```python
from build123d import *

# Parameters (mm, degrees)
F0_R     = 14.75
F1_DEPTH = 20
F3_DEPTH = 17.53955
F4_DEPTH = 74
F6_DEPTH = 19
F7_W     = 3.96875
F7_H     = 17.4625
F8_DEPTH = 20.001


with BuildPart() as f1:
    # F0 (on Top) → F1 (new body)
    with BuildSketch(Plane.XY):
        Circle(F0_R)
    extrude(amount=F1_DEPTH)

    # F2 (on face) → F3 (join)
    with BuildSketch(Plane(origin=(0, 0, 0), x_dir=(1, 0, 0), z_dir=(0, 0, -1))):
        with BuildLine():
            Line((0, -14.75), (0, -17.8051246337))
            Line((0, -17.8051246337), (14.75, -17.8051246337))
            Line((14.75, -17.8051246337), (14.75, 0))
            ThreePointArc((14.75, 0), (10.4298250225, -10.4298250225), (0, -14.75))
        make_face()
        with BuildLine():
            Line((-14.75, -17.8051246337), (0, -17.8051246337))
            Line((0, -17.8051246337), (0, -14.75))
            ThreePointArc((0, -14.75), (-10.4298250225, -10.4298250225), (-14.75, 0))
            Line((-14.75, 0), (-14.75, -17.8051246337))
        make_face()
        with BuildLine():
            ThreePointArc((-14.75, 0), (-10.4298250225, -10.4298250225), (0, -14.75))
            Line((0, -14.75), (0, 0))
            Line((0, 0), (-14.75, 0))
        make_face()
        with BuildLine():
            Line((0, 0), (0, -14.75))
            ThreePointArc((0, -14.75), (10.4298250225, -10.4298250225), (14.75, 0))
            Line((14.75, 0), (0, 0))
        make_face()
        Polygon((14.75, -17.8051246337), (0, -17.8051246337), (-14.75, -17.8051246337), (-14.75, -37.8051246337), (14.75, -37.8051246337), align=None)
    extrude(amount=-F3_DEPTH)

    # F2 (on face) → F4 (join)
    with BuildSketch(Plane(origin=(0, 0, 0), x_dir=(1, 0, 0), z_dir=(0, 0, -1))):
        Polygon((14.75, -17.8051246337), (0, -17.8051246337), (-14.75, -17.8051246337), (-14.75, -37.8051246337), (14.75, -37.8051246337), align=None)
    extrude(amount=F4_DEPTH)

    # F5 (on face) → F6 (cut)
    with BuildSketch(Plane.XY.offset(20)):
        with BuildLine():
            Line((2, -1.5), (2, 1.5))
            ThreePointArc((2, 1.5), (-2.5, 0), (2, -1.5))
        make_face()
    extrude(amount=-F6_DEPTH, mode=Mode.SUBTRACT)

    # F7 (on face) → F8 (cut, through all)
    with BuildSketch(Plane.XZ.offset(-17.8051246337)):
        with Locations((5.159375, -34.33125)):
            Rectangle(F7_W, F7_H)
        with Locations((-5.159375, -34.33125)):
            Rectangle(F7_W, F7_H)
    extrude(amount=-F8_DEPTH, mode=Mode.SUBTRACT)


solid = f1.part
```
Could you check a few things on this model? Use its own coordinates, in mm. A direction names the side the tool comes from. Give positions to 0.01 mm unless a question says otherwise; leave off trailing zeros. Write each loop counter-clockwise with the first axis right and the second up, starting at its lowest first coordinate (ties: lowest second). Pieces come first, ordered by that corner, then holes. Notation, with made-up numbers: (-39, -14) - (4, -14) arc R27 cw to (4, 2) - close; hole circle Ø8 at (69.25, -18). An arc over 180 degrees is marked (long way). One line per item, written item: value. Start each with the question number.
Item 1: Imagine slicing it at C-C, the plane x = 0. List the corners of the cut face in (y, z) for me, and give its area (3 significant figures).
Item 2: I'm going to push flat-ended pins straight in: pin 1 (10 mm diameter, centred on x = 4.5, z = 8.5, fed in from -Y); pin 2 (1 mm diameter, centred on x = -4, y = 24.5, fed in from +Z); pin 3 (6 mm diameter, centred on x = 4.5, z = -59.5, fed in from -Y); pin 4 (5 mm diameter, centred on y = -3.5, z = -4.5, fed in from +X). Where does each tip first touch, or does it pass through?
Item 3: Imagine slicing it at A-A, the plane z = -30. List the corners of the cut face in (x, y) for me (3 decimals).
Item 4: If we mould it in two halves opening along Z, with no side actions, what happens to faces 4 (the face through (-3.175, 28, -34)), 5 (the face through (14.75, 23, -17)), 6 (the face through (0, 23, 17.54))? For each: +Z half, -Z half, draft (parallel to the pull), parting line (faces both ways), or undercut.
Item 5: Please list where these lines run through material, in increasing order: line 1 (X direction, y = 27.5, z = -27) (3 decimals); line 2 (Y direction, x = 0, z = 7.25); line 3 (Z direction, x = -1, y = 18). Write a range as from..to.
Item 6: Imagine slicing it at D-D, the plane z = 12. List the corners of the cut face in (x, y) for me.
Item 7: Imagine slicing it at B-B, the plane y = 31.5. Give the number of separate pieces and of enclosed holes in the cut face, and give its area (3 significant figures).
Item 8: Which directions (+Z, -Z, +X, -X, +Y, -Y) give clear straight access to the entire face, cutting with the end or side of a thin tool? Please do faces 1 (the face through (-2.5, 0.1, 10.6)), 2 (the face through (0, 17.805, -36)), 3 (the face through (7.144, 28, -34)).
Geometry says:
1. outline: (-14.75, 0) - (17.81, 0) - (17.81, -74) - (37.81, -74) - (37.81, 17.54) - (14.75, 17.54) - (14.75, 20) - (2.5, 20) - (2.5, 1) - (-2.5, 1) - (-2.5, 20) - (-14.75, 20) - close
1. area: 2,380 mm^2
2. pin 1: y = -14.75
2. pin 2: z = 17.54
2. pin 3: y = 17.81
2. pin 4: through
3. outline: (-14.75, 17.805) - (-7.144, 17.805) - (-7.144, 37.805) - (-14.75, 37.805) - close; (-3.175, 17.805) - (3.175, 17.805) - (3.175, 37.805) - (-3.175, 37.805) - close; (7.144, 17.805) - (14.75, 17.805) - (14.75, 37.805) - (7.144, 37.805) - close
4. face 4: undercut
4. face 5: draft
4. face 6: +Z half
5. line 1: -14.75..-7.144, -3.175..3.175, 7.144..14.75
5. line 2: -14.75..-2.5, 2.5..37.81
5. line 3: -74..17.54
6. outline: (-14.75, 0) arc R14.75 ccw to (14.75, 0) - (14.75, 37.81) - (-14.75, 37.81) - close; hole (2, -1.5) - (2, 1.5) arc R2.5 ccw (long way) to start
7. separate pieces: 1
7. enclosed holes: 2
7. area: 2,560 mm^2
8. face 1: +Z
8. face 2: -Z, +X, -X, -Y
8. face 3: +Y, -Y
